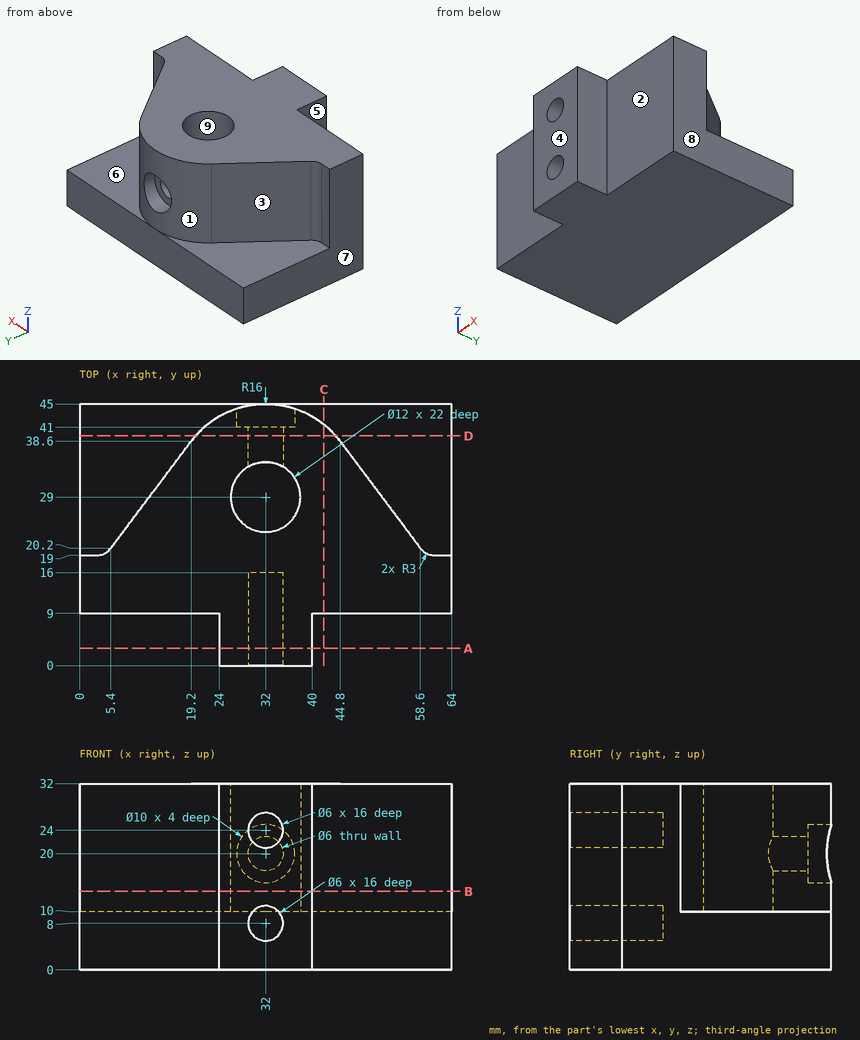
Can you work these out from the drawing? Everything is in mm from the part's minimum corner. A direction names the side the tool comes from. Round coordinates to 2 decimals unless told otherwise and drop trailing zeros. Loops run counter-clockwise (first coordinate to the right, second up) from the corner with the lowest first, then second, coordinate; pieces in that order, holes last. Notation, with made-up numbers: M -26,18 L -1,18 A12 cw -1,36 Z; hole C 87,-7.5 d11. An arc over 180 degrees is marked long. Answer in a Markdown table with one row per item.
1. If we section it at C-C, the plane x = 42: Please give me the cut outline in (y, z), plus the area to 3 significant figures.
Established:
| item | result |
|---|---|
| outline | M 9,0 L 45,0 L 45,10 L 41.49,10 L 41.49,32 L 9,32 Z |
| area | 1,070 mm² |
2. I'm going to push flat-ended pins straight in: pin 1 Ø4 at (x, z) = (36.5, 20) entering from +Y; pin 2 Ø7 at (y, z) = (5, 10.5) entering from -X; pin 3 Ø1.8 at (x, z) = (31.5, 6.5) entering from -Y. Where does each tip first touch, or does it pass through?
Established:
| item | result |
|---|---|
| pin 1 | y = 44.33 |
| pin 2 | x = 24 |
| pin 3 | y = 16 |
3. If we section it at A-A, the plane y = 3: Please give me the cut outline in (x, z), plus the area to 3 significant figures.
Established:
| item | result |
|---|---|
| outline | M 24,0 L 40,0 L 40,32 L 24,32 Z; hole C 32,8 d6; hole C 32,24 d6 |
| area | 455 mm² |
4. Please list where these lines run through material, in increasing order: line 1 (Z direction, x = 32, y = 8.5); line 2 (Y direction, x = 32, z = 29); line 3 (Z direction, x = 32, y = 36.75). Write a range as from..to.
Established:
| item | result |
|---|---|
| line 1 | 0..5, 11..21, 27..32 |
| line 2 | 0..23, 35..45 |
| line 3 | 0..17, 23..32 |
5. On a 3-axis mill with a long thin cutter (end or side, diameter ignored), from which of +Z, -Z, +X, -X, +Y, -Y can I reach the whole of each face in a straight line? I mean the marked faces 1, 2, 3, 4 and 5. Say none if no direction works.
Established:
| item | result |
|---|---|
| face 1 | +Z, +Y |
| face 2 | +Z, -Z, +X, -Y |
| face 3 | +Z, -X, +Y |
| face 4 | +Z, -Z, +X, -X, -Y |
| face 5 | +Z, -Z, -X, -Y |
6. If we section it at B-B, the plane z = 13.5: Please give me the cut outline in (x, y).
Established:
| item | result |
|---|---|
| outline | M 0,9 L 24,9 L 24,0 L 40,0 L 40,9 L 64,9 L 64,19 L 61,19 A3 cw 58.6,20.2 L 44.8,38.6 A16 ccw 19.2,38.6 L 5.4,20.2 A3 cw 3,19 L 0,19 Z; hole C 32,29 d12 |
7. Thinking about a two-plate mould opening in X: for the marked faces 6, 7, 8 and 9, which applies, pulls with the +X half, pulls with the -X half, needs draft (parallel to the pull), parting line crosses it, or undercut?
Established:
| item | result |
|---|---|
| face 6 | needs draft |
| face 7 | pulls with the -X half |
| face 8 | pulls with the +X half |
| face 9 | undercut |
8. If we section it at D-D, the plane y = 39.5: Please give me the cut outline in (x, z).
Established:
| item | result |
|---|---|
| outline | M 0,0 L 64,0 L 64,10 L 44.07,10 L 44.07,32 L 19.93,32 L 19.93,10 L 0,10 Z; hole C 32,20 d6 |
